Can you work these out from the drawing? Everything is in mm from the part's minimum corner. A direction names the side the tool comes from. Round coordinates to 2 decimals unless told otherwise and drop trailing zeros. Write each loop counter-clockwise with the first axis right and the second up, starting at its lowest first coordinate (ties: lowest second). Pieces come first, ordered by that corner, then holes. Notation, with made-up numbers: (62, -36) - (88, -36) arc R17 cw to (88, -24) - close; hole circle Ø7 at (28, -26.75). An arc over 180 degrees is marked (long way). Write each question's results on one line, items separated by ' | '. Start each with the question number.
(1) Imagine slicing it at C-C on z = 10. Write out the boundary of the cut face in (x, y).
(2) Please list where these lines run through material, in increasing order: line 1 (X direction, y = 5.25, z = 48.5) (1 decimal); line 2 (Z direction, x = 4.5, y = 4.5) (1 decimal); line 3 (Z direction, x = 1, y = 20.75). Write a range as [from, to].
(3) On a 3-axis mill with a long thin cutter (end or side, diameter ignored), from which of +Z, -Z, +X, -X, +Y, -Y can I reach the whole of each face in a straight line? I mean the marked faces 1, 2 and 3. Say none if no direction works.
(4) Imagine slicing it at D-D on y = 5. Write out the boundary of the cut face in (x, z), then the cut area to 3 significant figures.
(5) Imagine slicing it at A-A on x = 5. State how many separate pieces and enclosed holes the cut face has, then the cut area to 3 significant figures.
(6) For P1, Ø5, axis at x = 4, y = 13.5, coming from the -Z side; P2, Ø4, axis at x = 5, z = 48.63, coming from the +Y side; P3, Ø2, axis at x = 5, y = 5, coming from the -Z side, each with a flat end and sliding along its axis, tell me the tip position at first contact or that it passes through.
(7) Imagine slicing it at B-B on y = 9. Write out the boundary of the cut face in (x, z).
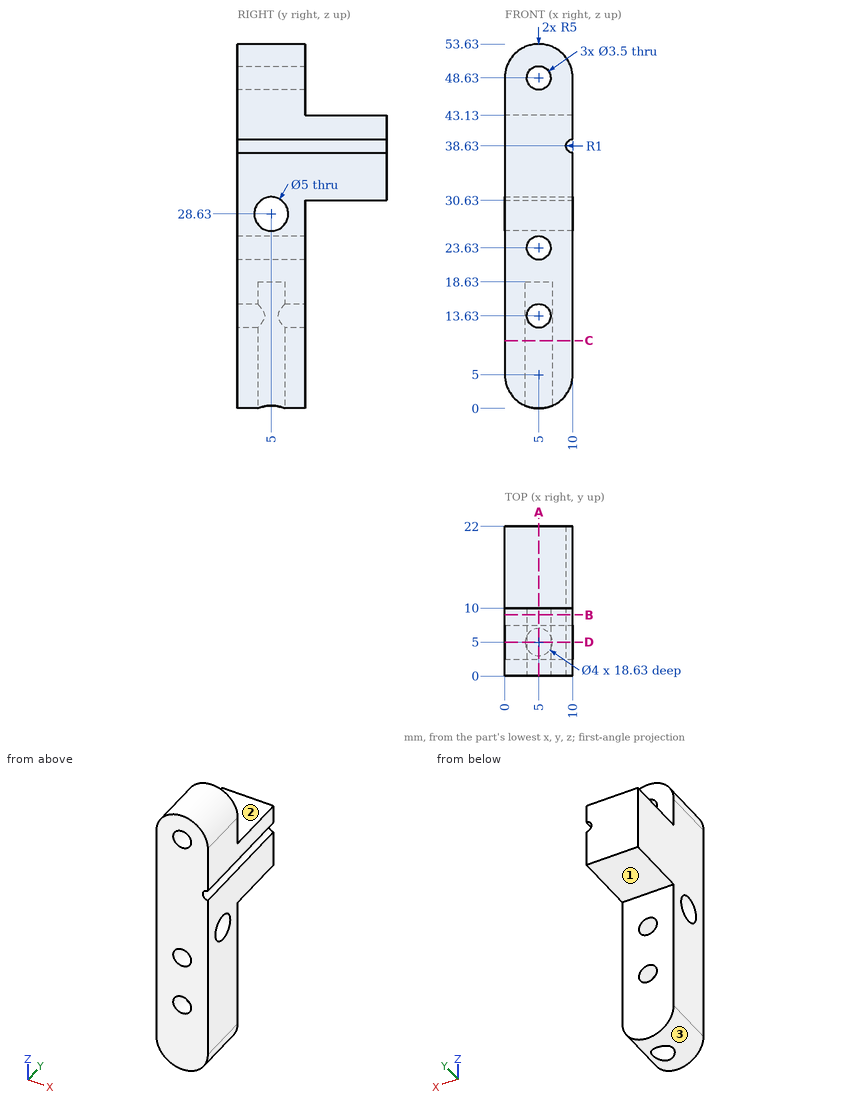
Response:
1) outline: (0, 0) - (10, 0) - (10, 10) - (0, 10) - close; hole circle Ø4 at (5, 5)
2) line 1: [0, 3.3], [6.7, 10] | line 2: [18.6, 22], [25.3, 26.2], [31.1, 47], [50.3, 53.6] | line 3: [30.63, 43.13]
3) face 1: -Z, +X, -X, +Y | face 2: +Z, +X, -X, +Y | face 3: -Z, +Y, -Y
4) outline: (0, 5) arc R5 ccw to (3, 0.42) - (3, 18.63) - (7, 18.63) - (7, 0.42) arc R5 ccw to (10, 5) - (10, 26.13) - (0, 26.13) - close; (0, 31.13) - (10, 31.13) - (10, 37.63) arc R1 cw to (10, 39.63) - (10, 48.63) arc R5 ccw to (0, 48.63) - close; hole circle Ø3.5 at (5, 23.63); hole circle Ø3.5 at (5, 48.63) | area: 370 mm²
5) separate pieces: 5 | enclosed holes: 1 | area: 501 mm²
6) P1: z = 30.63 | P2: y = 10 | P3: z = 18.63
7) outline: (0, 5) arc R5 ccw to (10, 5) - (10, 37.63) arc R1 cw to (10, 39.63) - (10, 48.63) arc R5 ccw to (0, 48.63) - close; hole circle Ø3.5 at (5, 13.63); hole circle Ø3.5 at (5, 23.63); hole circle Ø3.5 at (5, 48.63)
